```python
from build123d import *

# Parameters (mm, degrees)
SKETCH1_W           = 5
SKETCH1_H           = 5
BOSS_EXTRUDE1_DEPTH = 141.3
SKETCH3_R           = 0.85
CUT_EXTRUDE2_DEPTH  = 142.41053709


with BuildPart() as part:
    # Sketch1 → Boss-Extrude1 (new body)
    with BuildSketch(Plane.XY):
        Rectangle(SKETCH1_W, SKETCH1_H)
    extrude(amount=BOSS_EXTRUDE1_DEPTH)

    # Sketch3 → Cut-Extrude2 (cut, through all)
    with BuildSketch(Plane.XZ.offset(2.5)):
        with Locations(Location((0, 138.8, 0), (0, 0, 270))):
            Circle(SKETCH3_R)
        with Locations(Location((0, 2.5, 0), (0, 0, 90))):
            Circle(SKETCH3_R)
        with Locations(Location((0, 84.15, 0), (0, 0, 270))):
            Circle(SKETCH3_R)
        with Locations(Location((0, 57.15, 0), (0, 0, 90))):
            Circle(SKETCH3_R)
    extrude(amount=-CUT_EXTRUDE2_DEPTH, mode=Mode.SUBTRACT)


solid = part.part
```
Geometry check sheet. Reference: the model listing, model coordinates, mm. Give positions to 0.01 mm unless a question says otherwise; leave off trailing zeros. Loops run counter-clockwise (first coordinate to the right, second up) from the corner with the lowest first, then second, coordinate; pieces in that order, holes last. Notation, with made-up numbers: M 42,45 L 56,45 A3 ccw 56,50 Z; hole C 71,45 d3. An arc over 180 degrees is marked long. Answer as CSV lines item,"result".
Item 1: Cross-section at A-A on x = 0. Record the cut outline in (y, z), and give its area (4 significant figures).
Values:
outline,"M -2.5,0 L 2.5,0 L 2.5,1.65 L -2.5,1.65 Z; M -2.5,3.35 L 2.5,3.35 L 2.5,56.3 L -2.5,56.3 Z; M -2.5,58 L 2.5,58 L 2.5,83.3 L -2.5,83.3 Z; M -2.5,85 L 2.5,85 L 2.5,137.95 L -2.5,137.95 Z; M -2.5,139.65 L 2.5,139.65 L 2.5,141.3 L -2.5,141.3 Z"
area,"672.5 mm²"
Item 2: Depth check by flat-ended pin: P1, Ø1, axis at x = 0, z = 138.8, coming from the -Y side (3 decimals). Enter the tip coordinate at first touch or a pass-through.
Values:
P1,"passes through"
Item 3: Material ranges on line 1 (X direction, y = -0.85, z = 138.8); line 2 (Z direction, x = -0.7, y = -1.65), recorded low to high.
Values:
line 1,"x = -2.5 to -0.85, 0.85 to 2.5"
line 2,"z = 0 to 2.02, 2.98 to 56.67, 57.63 to 83.67, 84.63 to 138.32, 139.28 to 141.3"
